Geometry check sheet. Reference: the model listing, model coordinates, mm. A direction names the side the tool comes from. Give positions to 0.01 mm unless a question says otherwise; leave off trailing zeros. Order: outer loops, then holes, each group sorted by start corner. A loop starts at its lowest first (then second) coordinate and runs counter-clockwise, first axis right, second up. Notation, with made-up numbers: M -17,-6 L 32,-6 A15 ccw 32,-2 Z; hole C 22.5,56.25 d10. An arc over 180 degrees is marked long. Answer as CSV lines item,"result".
from build123d import *

# Parameters (mm, degrees)
SKETCH1_R               = 5.5
SKETCH1_R_2             = 2.58
BOSS_EXTRUDE1_DEPTH     = 72.14
SKETCH5_R               = 6.5785
BOSS_EXTRUDE2_DEPTH     = 12
SKETCH6_R               = 10.5
BOSS_EXTRUDE3_DEPTH     = 25
G1_4_TAPPED_HOLE2_D     = 11.8
G1_4_TAPPED_HOLE2_DEPTH = 20
G1_4_TAPPED_HOLE2_TIP   = 3.545077652
SKETCH15_R              = 2.5
BOSS_EXTRUDE4_DEPTH     = 18
M8_TAPPED_HOLE1_D       = 6.8
M8_TAPPED_HOLE1_DEPTH   = 79.14
M8_TAPPED_HOLE1_TIP     = 2.042926105
SKETCH18_R              = 4.5
CUT_EXTRUDE1_DEPTH      = 20


with BuildPart() as part:
    # Sketch1 → Boss-Extrude1 (new body)
    with BuildSketch(Plane(origin=(0, 0, 0), x_dir=(1, 0, 0), z_dir=(0, 1, 0))):
        with Locations(Location((0, 0, 0), (0, 0, 270))):
            Circle(SKETCH1_R)
        with Locations(Location((0, 0, 0), (0, 0, 270))):
            Circle(SKETCH1_R_2, mode=Mode.SUBTRACT)
    extrude(amount=BOSS_EXTRUDE1_DEPTH)

    # Sketch5 → Boss-Extrude2 (add)
    with BuildSketch(Plane(origin=(0, 72.14, 0), x_dir=(1, 0, 0), z_dir=(0, 1, 0))):
        with Locations(Location((0, 0, 0), (0, 0, 270))):
            Circle(SKETCH5_R)
    extrude(amount=BOSS_EXTRUDE2_DEPTH)

    # Sketch6 → Boss-Extrude3 (add)
    with BuildSketch(Plane(origin=(0, 84.14, 0), x_dir=(1, 0, 0), z_dir=(0, 1, 0))):
        with Locations(Location((0, 0, 0), (0, 0, 270))):
            Circle(SKETCH6_R)
    extrude(amount=BOSS_EXTRUDE3_DEPTH)

    # G1/4 Tapped Hole2
    with Locations(Plane(origin=(0, 109.14, 0), x_dir=(1, 0, 0), z_dir=(0, 1, 0))):
        with Locations((0, 0)):
            Hole(G1_4_TAPPED_HOLE2_D / 2, depth=G1_4_TAPPED_HOLE2_DEPTH)
            with Locations((0, 0, -(G1_4_TAPPED_HOLE2_DEPTH + G1_4_TAPPED_HOLE2_TIP / 2))):  # 118° drill point
                Cone(0, G1_4_TAPPED_HOLE2_D / 2, G1_4_TAPPED_HOLE2_TIP, mode=Mode.SUBTRACT)

    # Sketch15 → Boss-Extrude4 (add)
    with BuildSketch(Plane(origin=(0, 90.14, 0), x_dir=(-1, 0, 0), z_dir=(0, -1, 0))):
        with Locations(Location((0, 0, 0), (0, 0, 270))):
            Circle(SKETCH15_R)
    extrude(amount=BOSS_EXTRUDE4_DEPTH)

    # M8 Tapped Hole1
    with Locations(Plane(origin=(0, 90.14, 0), x_dir=(1, 0, 0), z_dir=(0, 1, 0))):
        with Locations((0, 0)):
            Hole(M8_TAPPED_HOLE1_D / 2, depth=M8_TAPPED_HOLE1_DEPTH)
            with Locations((0, 0, -(M8_TAPPED_HOLE1_DEPTH + M8_TAPPED_HOLE1_TIP / 2))):  # 118° drill point
                Cone(0, M8_TAPPED_HOLE1_D / 2, M8_TAPPED_HOLE1_TIP, mode=Mode.SUBTRACT)

    # Sketch18 → Cut-Extrude1 (cut)
    with BuildSketch(Plane.XY):
        with Locations(Location((0, 91.64, 0), (0, 0, 180))):
            Circle(SKETCH18_R)
    extrude(amount=CUT_EXTRUDE1_DEPTH, mode=Mode.SUBTRACT)


solid = part.part
(1) Section check B-B on y = 34. Enter the section's corners in (x, z), then the cut area to 3 significant figures.
The answers:
outline,"C 0,0 d11; hole C 0,0 d6.8"
area,"58.7 mm2"
(2) Gauge pin test, flat ends, axial feed: P1, Ø6, axis at y = 47.5, z = 7, coming from the +X side; P2, Ø8, axis at x = -8, y = 76, coming from the -Z side; P3, Ø3, axis at x = -5.5, y = 37, coming from the +Z side; P4, Ø4, axis at x = 0, z = 0, coming from the -Y side. Record the tip position at first contact, or that the pin passes through.
The answers:
P1,"stops at x = 3.77"
P2,"stops at z = -5.22"
P3,"stops at z = 3.77"
P4,"passes through"
(3) Section check D-D on x = 8.75. Enter the section's corners in (y, z), then the cut area to 3 significant figures.
The answers:
outline,"M 84.14,-5.8 L 109.14,-5.8 L 109.14,5.8 L 84.14,5.8 Z"
area,"290 mm2"
(4) Tool access check on faces 1 (the face through (-1.57, 5.18, -2.047)), 2 (the face through (0.59, 87.18, 7.41)), 3 (the face through (0.77, 99, -5.85)), 4 (the face through (-5, 109.14, 5)), 5 (the face through (-4, 72.14, -4)). Record the directions out of +Z, -Z, +X, -X, +Y, -Y that give a thin tool (end or side, any length) a straight path to the whole face; none if there is none.
The answers:
face 1,"+Y, -Y"
face 2,"+Z"
face 3,"+Y"
face 4,"+Z, -Z, +X, -X, +Y"
face 5,"-Y"
(5) Draft check along X on faces 6 (the face through (-2.52, 78.056, 6.077)), 7 (the face through (0, 88, -4)), 8 (the face through (5, 84.14, 5)). Enter one of: +X half, -X half, draft (parallel to the pull), parting line (faces both ways), or undercut.
The answers:
face 6,"parting line"
face 7,"undercut"
face 8,"draft"
(6) Material ranges on line 1 (Y direction, x = 0, z = 8.5); line 2 (Z direction, x = 0.5, y = 102); line 3 (X direction, y = 5, z = 0), recorded low to high.
The answers:
line 1,"y = 84.14 to 87.14, 96.14 to 109.14"
line 2,"z = -10.49 to -5.88, 5.88 to 10.49"
line 3,"x = -5.5 to -2.58, 2.58 to 5.5"
(7) Section check A-A on z = 0. Enter the section's corners in (x, y), then the cut area to 3 significant figures.
The answers:
outline,"M -10.5,84.14 L -6.58,84.14 L -6.58,72.14 L -5.5,72.14 L -5.5,0 L -2.58,0 L -2.58,10.51 L -3.4,11 L -3.4,87.64 L -5.9,89.14 L -5.9,109.14 L -10.5,109.14 Z; M 2.58,0 L 5.5,0 L 5.5,72.14 L 6.58,72.14 L 6.58,84.14 L 10.5,84.14 L 10.5,109.14 L 5.9,109.14 L 5.9,89.14 L 3.4,87.64 L 3.4,11 L 2.58,10.51 Z"
area,"648 mm2"
(8) Section check C-C on y = 81. Enter the section's corners in (x, z).
The answers:
outline,"C 0,0 d13.16; hole C 0,0 d6.8"
